from build123d import *

# Parameters (mm, degrees)
F0_R          = 14
F1_DEPTH      = 12.6
F2_R          = 12.9
F3_DEPTH      = 10.6
F5_DEPTH      = 10.6
F6_W          = 6
F6_H          = 9
F6_W_2        = 10
F6_H_2        = 8.5
F7_DEPTH      = 13
F7_DEPTH_BACK = 12
F9_DEPTH      = 6.6
F10_R         = 13.5
F11_DEPTH     = 12


with BuildPart() as f1:
    # F0 (on Top) → F1 (new body)
    with BuildSketch(Plane.XY):
        Circle(F0_R)
    extrude(amount=F1_DEPTH)

    # F2 (on face) → F3 (join)
    with BuildSketch(Plane.XY.offset(12.6)):
        Circle(F2_R)
    extrude(amount=F3_DEPTH)

    # F4 (on face) → F5 (cut)
    with BuildSketch(Plane.XY.offset(23.2)):
        with BuildLine():
            Line((19.0122332424, 15.1731111109), (11, 15.1731111109))
            Line((11, 15.1731111109), (11, 6.7386942355))
            ThreePointArc((11, 6.7386942355), (12.4159172033, 3.5007142128), (12.9, 0))
            ThreePointArc((12.9, 0), (12.4159172033, -3.5007142128), (11, -6.7386942355))
            Line((11, -6.7386942355), (11, -15.1731111109))
            Line((11, -15.1731111109), (19.0122332424, -15.1731111109))
            Line((19.0122332424, -15.1731111109), (19.0122332424, 15.1731111109))
        make_face()
        with BuildLine():
            Line((-11, -6.7386942355), (-11, 6.7386942355))
            ThreePointArc((-11, 6.7386942355), (-12.9, 0), (-11, -6.7386942355))
        make_face()
        with BuildLine():
            Line((-11, 6.7386942355), (-11, 13.9122297987))
            Line((-11, 13.9122297987), (-20.8380557597, 13.9122297987))
            Line((-20.8380557597, 13.9122297987), (-20.8380557597, -13.9122297987))
            Line((-20.8380557597, -13.9122297987), (-11, -13.9122297987))
            Line((-11, -13.9122297987), (-11, -6.7386942355))
            ThreePointArc((-11, -6.7386942355), (-12.9, 0), (-11, 6.7386942355))
        make_face()
        with BuildLine():
            ThreePointArc((12.9, 0), (12.4159172033, 3.5007142128), (11, 6.7386942355))
            Line((11, 6.7386942355), (11, -6.7386942355))
            ThreePointArc((11, -6.7386942355), (12.4159172033, -3.5007142128), (12.9, 0))
        make_face()
    extrude(amount=-F5_DEPTH, mode=Mode.SUBTRACT)

    # F6 (on face) → F7 (join, two sides)
    with BuildSketch(Plane.XY.offset(23.2)) as f7_sk:
        with Locations((-8, 0)):
            Rectangle(F6_W, F6_H)
        with Locations((0, 8.75)):
            Rectangle(F6_W_2, F6_H_2)
        Rectangle(F6_W_2, F6_H)
        with Locations((8, 0)):
            Rectangle(F6_W, F6_H)
        with Locations((0, -8.75)):
            Rectangle(F6_W_2, F6_H_2)
    extrude(amount=F7_DEPTH)
    extrude(f7_sk.sketch, amount=-F7_DEPTH_BACK)

    # F8 (on face) → F9 (join)
    with BuildSketch(Plane.XY.offset(12.6)):
        with BuildLine():
            Line((5, -13), (-5, -13))
            Line((-5, -13), (-5, -13.0766968306))
            ThreePointArc((-5, -13.0766968306), (0, -14), (5, -13.0766968306))
            Line((5, -13.0766968306), (5, -13))
        make_face()
        with BuildLine():
            ThreePointArc((5, 13.0766968306), (0, 14), (-5, 13.0766968306))
            Line((-5, 13.0766968306), (-5, 13))
            Line((-5, 13), (5, 13))
            Line((5, 13), (5, 13.0766968306))
        make_face()
    extrude(amount=F9_DEPTH)

    # F10 (on face) → F11 (cut)
    with BuildSketch(Plane(origin=(0, 0, 0), x_dir=(1, 0, 0), z_dir=(0, 0, -1))):
        Circle(F10_R)
    extrude(amount=-F11_DEPTH, mode=Mode.SUBTRACT)


solid = f1.part
Design review of the part built by this model. Coordinates are the model's own, in mm. A direction names the side the tool comes from. Round coordinates to 2 decimals unless told otherwise and drop trailing zeros. Loops run counter-clockwise (first coordinate to the right, second up) from the corner with the lowest first, then second, coordinate; pieces in that order, holes last. Notation, with made-up numbers: (-8.5, -4) -> (17.5, -4) arc R11 ccw to (17.5, 2) -> close; hole circle Ø3 at (-23.75, -16). An arc over 180 degrees is marked (long way). Use one line per item in the form item = value. Start each with the question number.
Q1. Wall thickness on line 1 along Y through (x, z) = (0, 5); line 2 along Z through (x, y) = (-2.75, -6.5): over which ranges is each line inside the solid? List them lowest first. Write a range as [from, to].
Q2. For pin 1 Ø4.5 at (y, z) = (-9.5, 25) entering from -X; pin 2 Ø6 at (x, z) = (-3, 23) entering from +Y; pin 3 Ø2 at (x, y) = (7.5, 6) entering from +Z, all flat-tipped, find the tip position at first contact; note any pin that passes through.
Q3. We need section A-A on z = 20.5. Give the boundary of the cut face in (x, y).
Q4. Machinability: for faces 1 (the face through (11.15, -0.91, 12.6)), 2 (the face through (-8.362, 9.823, 17.826)), 3 (the face through (0, -13, 28)), 4 (the face through (-8, -4.5, 30)), which of the approach directions +Z, -Z, +X, -X, +Y, -Y give a long, thin tool a straight path to every point of the face, cutting with its end or side? Answer none if there is none.
Q5. We need section C-C on x = -9.25. Give the boundary of the cut face in (y, z), then the cut area to 3 significant figures.
Q6. We need section B-B on y = 0. Give the boundary of the cut face in (x, z), then the cut area to 3 significant figures.
Q7. We need section D-D on z = 2.5. Give the boundary of the cut face in (x, y).
Calculated:
q1.line_1 = [-14, -13.5], [13.5, 14]
q1.line_2 = [12, 36.2]
q2.pin_1 = -10
q2.pin_2 = 13
q2.pin_3 = 23.2
q3.outline = (-11, -6.74) arc R12.9 ccw to (-5, -11.89) -> (-5, -13) -> (5, -13) -> (5, -11.89) arc R12.9 ccw to (11, -6.74) -> (11, 6.74) arc R12.9 ccw to (5, 11.89) -> (5, 13) -> (-5, 13) -> (-5, 11.89) arc R12.9 ccw to (-11, 6.74) -> close
q4.face_1 = +Z, +X
q4.face_2 = +Z, -X, +Y
q4.face_3 = +Z, +X, -X, -Y
q4.face_4 = +Z, -X, -Y
q5.outline = (-10.51, 0) -> (-9.83, 0) -> (-9.83, 12) -> (9.83, 12) -> (9.83, 0) -> (10.51, 0) -> (10.51, 12.6) -> (8.99, 12.6) -> (8.99, 23.2) -> (4.5, 23.2) -> (4.5, 36.2) -> (-4.5, 36.2) -> (-4.5, 23.2) -> (-8.99, 23.2) -> (-8.99, 12.6) -> (-10.51, 12.6) -> close
q5.area = 336 mm²
q6.outline = (-14, 0) -> (-13.5, 0) -> (-13.5, 12) -> (13.5, 12) -> (13.5, 0) -> (14, 0) -> (14, 12.6) -> (11, 12.6) -> (11, 36.2) -> (-11, 36.2) -> (-11, 12.6) -> (-14, 12.6) -> close
q6.area = 548 mm²
q7.outline = circle Ø28 at (0, 0); hole circle Ø27 at (0, 0)
